Part print with two shaded views. Sizes in mm from the minimum x, y, z corner. Round coordinates to 2 decimals unless told otherwise and drop trailing zeros. Order: outer loops, then holes, each group sorted by start corner. A loop starts at its lowest first (then second) coordinate and runs counter-clockwise, first axis right, second up. Notation, with made-up numbers: (2, 52) - (19, 52) arc R33 cw to (19, 82) - close; hole circle Ø3 at (32.25, -13). An arc over 180 degrees is marked (long way). Use one line per item in the form item = value.
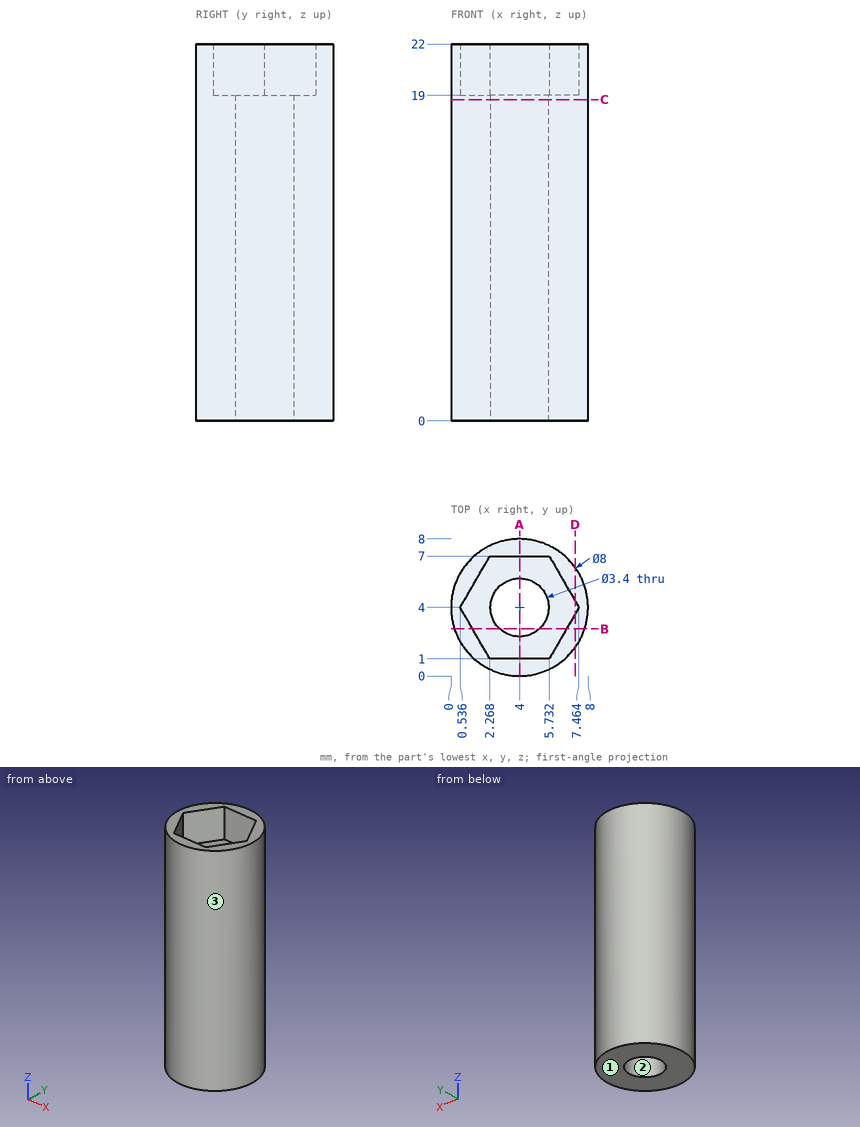
(1) Pull direction X, two halves, no side cores. Call the marked faces 1, 2 and 3: released by +X, released by -X, zero draft, split by the parting line, or undercut.
Report:
face_1 = zero draft
face_2 = undercut
face_3 = split by the parting line
(2) Pin check, flat tips, straight feed: pin 1 (1.5 mm diameter, centred on x = 2, z = 7, fed in from +Y); pin 2 (1 mm diameter, centred on x = 2.5, z = 16.5, fed in from +Y); pin 3 (4.5 mm diameter, centred on x = 4, y = 4, fed in from +Z). Stop position of each tip, or through.
Report:
pin_1 = 7.8
pin_2 = 7.87
pin_3 = 19
(3) Probe probe 1 along Y at (x, z) = (4, 11.25); probe 2 along X at (y, z) = (2, 2.25); probe 3 along X at (y, z) = (5.5, 16.5). List the from-to ranges inside material, lowest first. Write a range as [from, to].
Report:
probe_1 = [0, 2.3], [5.7, 8]
probe_2 = [0.54, 7.46]
probe_3 = [0.29, 3.2], [4.8, 7.71]
(4) Slice it at C-C on z = 18.75. Give the cut face in (x, y).
Report:
outline = circle Ø8 at (4, 4); hole circle Ø3.4 at (4, 4)
(5) Slice it at A-A on x = 4. Give the cut face in (y, z), then the cut area to 3 significant figures.
Report:
outline = (0, 0) - (2.3, 0) - (2.3, 19) - (1, 19) - (1, 22) - (0, 22) - close; (5.7, 0) - (8, 0) - (8, 22) - (7, 22) - (7, 19) - (5.7, 19) - close
area = 93.4 mm2
(6) Slice it at B-B on y = 2.75. Give the cut face in (x, z), then the cut area to 3 significant figures.
Report:
outline = (0.2, 0) - (2.85, 0) - (2.85, 19) - (1.26, 19) - (1.26, 22) - (0.2, 22) - close; (5.15, 0) - (7.8, 0) - (7.8, 22) - (6.74, 22) - (6.74, 19) - (5.15, 19) - close
area = 107 mm2
(7) Slice it at D-D on x = 7.25. Give the cut face in (y, z).
Report:
outline = (1.67, 0) - (6.33, 0) - (6.33, 22) - (4.37, 22) - (4.37, 19) - (3.63, 19) - (3.63, 22) - (1.67, 22) - close
